from build123d import *

# Parameters (mm, degrees)
BOSS_EXTRUDE1_DEPTH = 6
BOSS_EXTRUDE2_DEPTH = 21
BOSS_EXTRUDE3_START = 21
SKETCH1_6_W         = 20
SKETCH1_6_H         = 21.2
SKETCH1_6_R         = 3.05
BOSS_EXTRUDE3_DEPTH = 10.48


with BuildPart() as part:
    # Sketch1 → Boss-Extrude1 (new body)
    with BuildSketch(Plane(origin=(0, 0, 0), x_dir=(1, 0, 0), z_dir=(0, 1, 0))):
        Polygon((-37.5, 40.45), (-37.5, -24.85), (26, -24.85), (26, 40.45), (6, 40.45), (6, 35.45), (21, 35.45), (21, 19.85), (-21, 19.85), (-21, 35.45), (-17.5, 35.45), (-17.5, 40.45), align=None)
    extrude(amount=BOSS_EXTRUDE1_DEPTH)

    # Sketch1_5 → Boss-Extrude2 (add)
    with BuildSketch(Plane(origin=(0, 0, 0), x_dir=(1, 0, 0), z_dir=(0, 1, 0))):
        Polygon((-37.5, 40.45), (-37.5, -24.85), (26, -24.85), (26, 40.45), (6, 40.45), (6, 35.45), (21, 35.45), (21, 19.85), (21, -19.85), (-21, -19.85), (-21, 19.85), (-21, 35.45), (-17.5, 35.45), (-17.5, 40.45), align=None)
    extrude(amount=BOSS_EXTRUDE2_DEPTH)

    # Sketch1_6 → Boss-Extrude3 (add)
    with BuildSketch(Plane(origin=(0, 0, 0), x_dir=(1, 0, 0), z_dir=(0, 1, 0)).offset(BOSS_EXTRUDE3_START)):
        with Locations((-27.5, 51.05)):
            Rectangle(SKETCH1_6_W, SKETCH1_6_H)
        with Locations(Location((-27.5, 48.65, 0), (0, 0, 270))):
            Circle(SKETCH1_6_R, mode=Mode.SUBTRACT)
        with Locations((16, 51.05)):
            Rectangle(SKETCH1_6_W, SKETCH1_6_H)
        with Locations(Location((16, 48.65, 0), (0, 0, 270))):
            Circle(SKETCH1_6_R, mode=Mode.SUBTRACT)
    extrude(amount=-BOSS_EXTRUDE3_DEPTH)


solid = part.part
Could you check a few things on this model? Use its own coordinates, in mm. A direction names the side the tool comes from. Give positions to 0.01 mm unless a question says otherwise; leave off trailing zeros. Order: outer loops, then holes, each group sorted by start corner. A loop starts at its lowest first (then second) coordinate and runs counter-clockwise, first axis right, second up.
1. We'd pull the mould along Z, two halves only. Please class faces 4 (the flat face through (16, 5, -40.45)), 5 (the flat face through (-6, 10, 24.85)), 6 (the cylindrical face through (-29.356, 15.833, -51.07)): pulls with the +Z half, pulls with the -Z half, needs draft (parallel to the pull), parting line crosses it, or undercut.
2. Suppose I cut it at A-A (z = -24). List the corners of the cut face in (x, y) for me, plus the area to 4 significant figures.
3. I need wall thicknesses on L1, parallel to X at y = 15, z = -48.65; L2, parallel to X at y = 11.75, z = 4.5; L3, parallel to Z at x = 7, y = 4. Which ranges of each line are inside material? Lowest first, please.
4. Suppose I cut it at C-C (x = 16). List the corners of the cut face in (y, z) for me, plus the area to 3 significant figures.
5. For faces 1 (the flat face through (-21, 13, -7)), 2 (the flat face through (6, 15, -46)), 3 (the flat face through (0, 3, -19.85)), which set-ups out of +Z, -Z, +X, -X, +Y, -Y let a thin tool reach every point of the face, with its end or its side?
6. Suppose I cut it at D-D (z = -48.65). List the corners of the cut face in (x, y) for me, plus the area to 3 significant figures.
7. Will these pins go through, and if not, where does the flat tip stop? P1, Ø10, axis at x = 3, z = -44, coming from the +Y side; P2, Ø3.5, axis at x = 16, z = -48.65, coming from the +Y side; P3, Ø5.5, axis at x = 18.5, y = 5, coming from the -Z side; P4, Ø4.5, axis at x = -9, y = 10, coming from the -Z side.
8. Suppose I cut it at B-B (x = -27.5). List the corners of the cut face in (y, z) for me.
Solved:
1. face 4: pulls with the -Z half
1. face 5: pulls with the +Z half
1. face 6: undercut
2. outline: (-37.5, 0) - (-21, 0) - (-21, 21) - (-37.5, 21) - close; (21, 0) - (26, 0) - (26, 21) - (21, 21) - close
2. area: 451.5 mm2
3. L1: x = -37.5 to -30.55, -24.45 to -17.5, 6 to 12.95, 19.05 to 26
3. L2: x = -37.5 to -21, 21 to 26
3. L3: z = -40.45 to -35.45, -19.85 to 24.85
4. outline: (0, -40.45) - (10.52, -40.45) - (10.52, -45.6) - (21, -45.6) - (21, -35.45) - (0, -35.45) - close; (0, -19.85) - (6, -19.85) - (6, 19.85) - (21, 19.85) - (21, 24.85) - (0, 24.85) - close; (10.52, -61.65) - (21, -61.65) - (21, -51.7) - (10.52, -51.7) - close
4. area: 606 mm2
5. face 1: +Y
5. face 2: -Z, +Y, -Y
5. face 3: +Y, -Y
6. outline: (-37.5, 10.52) - (-30.55, 10.52) - (-30.55, 21) - (-37.5, 21) - close; (-24.45, 10.52) - (-17.5, 10.52) - (-17.5, 21) - (-24.45, 21) - close; (6, 10.52) - (12.95, 10.52) - (12.95, 21) - (6, 21) - close; (19.05, 10.52) - (26, 10.52) - (26, 21) - (19.05, 21) - close
6. area: 291 mm2
7. P1: stops at y = 21
7. P2: passes through
7. P3: stops at z = -40.45
7. P4: stops at z = 19.85
8. outline: (0, -40.45) - (10.52, -40.45) - (10.52, -45.6) - (21, -45.6) - (21, 24.85) - (0, 24.85) - close; (10.52, -61.65) - (21, -61.65) - (21, -51.7) - (10.52, -51.7) - close
